```python
from build123d import *

# Parameters (mm, degrees)
CYLINDER006_R     = 2
CYLINDER006_DEPTH = 10
BOX005_W          = 8
BOX005_H          = 8
BOX005_DEPTH      = 10
FILLET002_R       = 2
CYLINDER007_R     = 2
CYLINDER007_DEPTH = 10
BOX006_W          = 8
BOX006_H          = 8
BOX006_DEPTH      = 10
FILLET003_R       = 2
PAD002_DEPTH      = 5
BOX002_W          = 19
BOX002_H          = 19
BOX002_DEPTH      = 10


with BuildPart() as cylinder006:
    # Cylinder006 → Cylinder006 (new body)
    with BuildSketch(Plane(origin=(4, 4, 0), x_dir=(1, 0, 0), z_dir=(0, 0, 1))):
        Circle(CYLINDER006_R)
    extrude(amount=CYLINDER006_DEPTH)


with BuildPart() as fillet002:
    # Box005 → Box005 (new body)
    with BuildSketch(Plane.XY):
        with Locations((4, 4)):
            Rectangle(BOX005_W, BOX005_H)
    extrude(amount=BOX005_DEPTH)

    # Cut006: cut Cylinder006
    add(cylinder006.part, mode=Mode.SUBTRACT)


with BuildPart() as fillet002_1:
    # Cut006 placement: moved
    add(fillet002.part.moved(Location((30, -10, 0))))

    # Fillet002
    fillet002_edges = [fillet002_1.edges().sort_by_distance(p)[0] for p in [
        (30, -10, 5),
        (38, -10, 5),
    ]]
    fillet(fillet002_edges, radius=FILLET002_R)


with BuildPart() as fillet002_2:
    # Fillet002 placement: moved
    add(fillet002_1.part.moved(Location((40, 0, 0))))


with BuildPart() as cylinder007:
    # Cylinder007 → Cylinder007 (new body)
    with BuildSketch(Plane(origin=(4, 4, 0), x_dir=(1, 0, 0), z_dir=(0, 0, 1))):
        Circle(CYLINDER007_R)
    extrude(amount=CYLINDER007_DEPTH)


with BuildPart() as fillet003:
    # Box006 → Box006 (new body)
    with BuildSketch(Plane.XY):
        with Locations((4, 4)):
            Rectangle(BOX006_W, BOX006_H)
    extrude(amount=BOX006_DEPTH)

    # Cut007: cut Cylinder007
    add(cylinder007.part, mode=Mode.SUBTRACT)


with BuildPart() as fillet003_1:
    # Cut007 placement: moved
    add(fillet003.part.moved(Location((45, 14, 0))))

    # Fillet003
    fillet003_edges = [fillet003_1.edges().sort_by_distance(p)[0] for p in [
        (45, 22, 5),
        (53, 22, 5),
    ]]
    fillet(fillet003_edges, radius=FILLET003_R)


with BuildPart() as fillet003_2:
    # Fillet003 placement: moved
    add(fillet003_1.part.moved(Location((36, 3, 0))))


with BuildPart() as obj1:
    # Sketch002 → Pad002 (new body)
    with BuildSketch(Plane(origin=(0, 0, 0), x_dir=(-1, 0, 0), z_dir=(0, 0, 1))):
        Polygon((-70, 0), (-70, -15.5), (-101.5, -8), (-101.5, 0), align=None)
    extrude(amount=PAD002_DEPTH)


with BuildPart() as obj1_1:
    # Body002 placement: moved
    add(obj1.part.moved(Location((0, 0, 5))))


with BuildPart() as obj2:
    # Box002 → Box002 (new body)
    with BuildSketch(Plane(origin=(70, -2, 0), x_dir=(1, 0, 0), z_dir=(0, 0, 1))):
        with Locations((9.5, 9.5)):
            Rectangle(BOX002_W, BOX002_H)
    extrude(amount=BOX002_DEPTH)

    # Cut002: cut obj1
    add(obj1_1.part, mode=Mode.SUBTRACT)

    # Fusion001: union Fillet002, Fillet003
    add(fillet002_2.part)
    add(fillet003_2.part)


solid = obj2.part
```
Geometry check sheet. Reference: the model listing, model coordinates, mm. A direction names the side the tool comes from. Give positions to 0.01 mm unless a question says otherwise; leave off trailing zeros. Order: outer loops, then holes, each group sorted by start corner. A loop starts at its lowest first (then second) coordinate and runs counter-clockwise, first axis right, second up. Notation, with made-up numbers: (57, 44.25) - (80, 44.25) arc R24 ccw to (80, 83.25) - close; hole circle Ø11 at (-29, 27.25). An arc over 180 degrees is marked (long way). Write item = value, one per line. Start each with the question number.
1) Scan lines: L1, parallel to Y at x = 74, z = 2; L2, parallel to Y at x = 85, z = 7.75; L3, parallel to Z at x = 77, y = 7. Record each from-to range of solid material in increasing order.
2) Section check C-C (z = 3.25). Enter the section's corners in (x, y).
3) Section check A-A (y = 21). Enter the section's corners in (x, z), then the cut area to 3 significant figures.
4) Section check B-B (z = 6.25). Enter the section's corners in (x, y), then the cut area to 3 significant figures.
5) Section check D-D (x = 74). Enter the section's corners in (y, z), then the cut area to 3 significant figures.
6) Draft check along X on faces 1 (the cylindrical face through (88.4, 24.43, 5.07)), 2 (the cylindrical face through (75.908, -5.399, 4.93)), 3 (the flat face through (79, 8, 0)). Enter one of: released by +X, released by -X, zero draft, split by the parting line, or undercut.
7) Access from +Z, -Z, +X, -X, +Y, -Y to the whole of each face (thin tool, end or side, straight path). Record for faces 4 (the flat face through (83, -2, 5)), 5 (the flat face through (75, 17, 5)), 6 (the flat face through (79.37, 13.27, 7.46)), 7 (the cylindrical face through (86.908, 21.601, 4.93)), 8 (the flat face through (80, 0, 7)).
8) Gauge pin test, flat ends, axial feed: pin 1 Ø3 at (y, z) = (-6.5, 5.5) entering from +X; pin 2 Ø1.5 at (x, z) = (79, 7.5) entering from +Y. Record the tip position at first contact, or that the pin passes through.
Geometry check:
q1.L1 = -10 to -8, -4 to 17
q1.L2 = -2 to 0, 11.93 to 19, 23 to 25
q1.L3 = 0 to 5
q2.outline = (70, -8) arc R2 ccw to (72, -10) - (76, -10) arc R2 ccw to (78, -8) - (78, -2) - (89, -2) - (89, 23) arc R2 ccw to (87, 25) - (83, 25) arc R2 ccw to (81, 23) - (81, 17) - (70, 17) - close; hole circle Ø4 at (74, -6); hole circle Ø4 at (85, 21)
q3.outline = (81, 0) - (83, 0) - (83, 10) - (81, 10) - close; (87, 0) - (89, 0) - (89, 10) - (87, 10) - close
q3.area = 40.0 mm2
q4.outline = (70, -8) arc R2 ccw to (72, -10) - (76, -10) arc R2 ccw to (78, -8) - (78, -2) - (89, -2) - (89, 0) - (70, 0) - close; (70, 15.5) - (89, 10.98) - (89, 23) arc R2 ccw to (87, 25) - (83, 25) arc R2 ccw to (81, 23) - (81, 17) - (70, 17) - close; hole circle Ø4 at (74, -6); hole circle Ø4 at (85, 21)
q4.area = 209 mm2
q5.outline = (-10, 0) - (-8, 0) - (-8, 10) - (-10, 10) - close; (-4, 0) - (17, 0) - (17, 10) - (14.55, 10) - (14.55, 5) - (0, 5) - (0, 10) - (-4, 10) - close
q5.area = 157 mm2
q6.face_1 = released by +X
q6.face_2 = undercut
q6.face_3 = zero draft
q7.face_4 = +Z, -Z, +X, -Y
q7.face_5 = +Z, -Z, -X, +Y
q7.face_6 = +Z, -X
q7.face_7 = +Z, -Z
q7.face_8 = +Z, +X, -X
q8.pin_1 = 78
q8.pin_2 = 17
